Here's how the part is built. I have some questions about the finished solid (model axes, mm). Round coordinates to 2 decimals unless told otherwise and drop trailing zeros. Loops run counter-clockwise (first coordinate to the right, second up) from the corner with the lowest first, then second, coordinate; pieces in that order, holes last. Notation, with made-up numbers: M 4.5,15 L 60.5,15 A22 ccw 60.5,31 Z; hole C 14,80 d10. An arc over 180 degrees is marked long. Write each question's results on one line, items separated by ' | '. Start each with the question number.
```python
from build123d import *

# Parameters (mm, degrees)
BOSS_EXTRUDE3_DEPTH              = 1.27
SKETCH4_W                        = 107.901987654
SKETCH4_H                        = 12.7
CUT_EXTRUDE1_DEPTH               = 1
CUT_EXTRUDE1_DEPTH_BACK          = 3.54
F_17_64_0_26563_DIAMETER_HOLE1_D = 6.747002


with BuildPart() as part:
    # Sketch2 → Boss-Extrude3 (new body, symmetric)
    with BuildSketch(Plane.XY):
        Polygon((-95.25, -25.4), (-95.25, 25.4), (0, 38.1), (0, -38.1), align=None)
    extrude(amount=BOSS_EXTRUDE3_DEPTH, both=True)

    # Sketch4 → Cut-Extrude1 (cut, two sides)
    with BuildSketch(Plane.XY.offset(1.27)) as cut_extrude1_sk:
        with Locations((-53.950993827, 31.75)):
            Rectangle(SKETCH4_W, SKETCH4_H)
    extrude(amount=CUT_EXTRUDE1_DEPTH, mode=Mode.SUBTRACT)
    extrude(cut_extrude1_sk.sketch, amount=-CUT_EXTRUDE1_DEPTH_BACK, mode=Mode.SUBTRACT)

    # 17/64 (0.26563) Diameter Hole1 (through all)
    with Locations(Plane.XY.offset(1.27)):
        with Locations((-82.55, 12.7), (-82.55, -12.7), (-12.7, -25.4), (-12.7, 12.7)):
            Hole(F_17_64_0_26563_DIAMETER_HOLE1_D / 2)


solid = part.part
```
1. For pin 1 (4 mm diameter, centred on x = -12.7, y = 12.7, fed in from +Z), with a flat end and sliding along its axis, tell me the tip position at first contact or that it passes through.
2. I want a section at A-A on y = -12.7. List the corners of the cut face in (x, z) for me.
3. I want a section at B-B on x = -82.55. List the corners of the cut face in (y, z) for me.
4. If we mould it in two halves opening along Y, with no side actions, what happens to faces 1 (the face through (-85.77, -11.69, -0.02)), 2 (the face through (0, -6, 0)), 3 (the face through (-12, -28.7, 0)), 4 (the face through (-48, 25.4, 0))? For each: released by +Y, released by -Y, zero draft, split by the parting line, or undercut.
5. I need wall thicknesses on line 1 along X through (y, z) = (14, 0.9); line 2 along Y through (x, z) = (-79.5, 0.4); line 3 along Y through (x, z) = (-12.7, 0.5). Which ranges of each line are inside material? Lowest first, please.
6. I want a section at C-C on y = 12.7. List the corners of the cut face in (x, z) for me.
7. I want a section at D-D on z = 0.75. List the corners of the cut face in (x, y) for me, plus the area to 3 significant figures.
Outcome:
1) pin 1: through
2) outline: M -95.25,-1.27 L -85.92,-1.27 L -85.92,1.27 L -95.25,1.27 Z; M -79.18,-1.27 L 0,-1.27 L 0,1.27 L -79.18,1.27 Z
3) outline: M -27.09,-1.27 L -16.07,-1.27 L -16.07,1.27 L -27.09,1.27 Z; M -9.33,-1.27 L 9.33,-1.27 L 9.33,1.27 L -9.33,1.27 Z; M 16.07,-1.27 L 25.4,-1.27 L 25.4,1.27 L 16.07,1.27 Z
4) face 1: undercut | face 2: zero draft | face 3: undercut | face 4: released by +Y
5) line 1: -95.25 to -85.66, -79.44 to -15.81, -9.59 to 0 | line 2: -27.5 to -14.14, -11.26 to 11.26, 14.14 to 25.4 | line 3: -36.41 to -28.77, -22.03 to 9.33, 16.07 to 25.4
6) outline: M -95.25,-1.27 L -85.92,-1.27 L -85.92,1.27 L -95.25,1.27 Z; M -79.18,-1.27 L -16.07,-1.27 L -16.07,1.27 L -79.18,1.27 Z; M -9.33,-1.27 L 0,-1.27 L 0,1.27 L -9.33,1.27 Z
7) outline: M -95.25,-25.4 L 0,-38.1 L 0,25.4 L -95.25,25.4 Z; hole C -82.55,-12.7 d6.75; hole C -82.55,12.7 d6.75; hole C -12.7,-25.4 d6.75; hole C -12.7,12.7 d6.75 | area: 5,300 mm2
